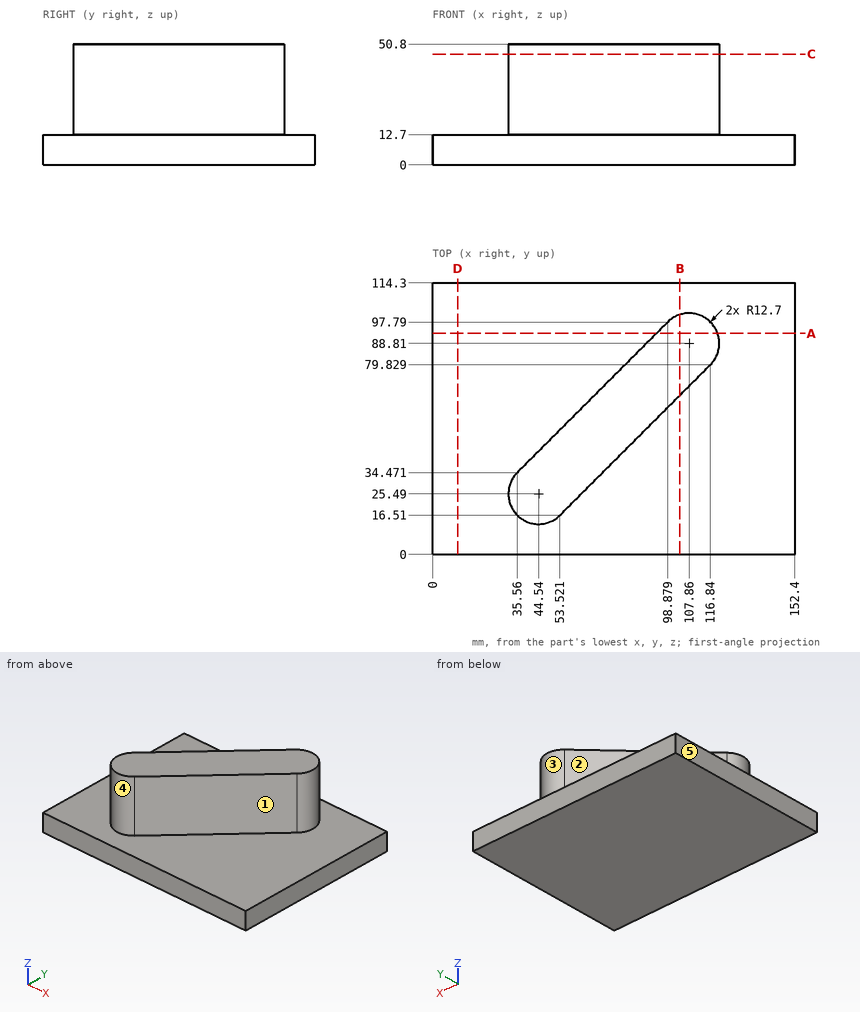
Job drawing, mm, ordinate dimensions from the low corner. One solid piece. A direction names the side the tool comes from. Round coordinates to 2 decimals unless told otherwise and drop trailing zeros. Order: outer loops, then holes, each group sorted by start corner. A loop starts at its lowest first (then second) coordinate and runs counter-clockwise, first axis right, second up. Notation, with made-up numbers: (42.25, 25) -> (67.25, 25) arc R33 ccw to (67.25, 58) -> close; hole circle Ø5 at (75, 52.25). An arc over 180 degrees is marked (long way). Write item = value, one per line.
(1) Cut at B-B (x = 104). Write the cut outline in (y, z).
Answers follow:
outline = (0, 0) -> (114.3, 0) -> (114.3, 12.7) -> (100.91, 12.7) -> (100.91, 50.8) -> (66.99, 50.8) -> (66.99, 12.7) -> (0, 12.7) -> close
(2) 3-axis set-ups, long thin cutter, end or side, ignore diameter. For the marked faces 4 and 5: which of +Z, -Z, +X, -X, +Y, -Y reach the whole face in a straight line?
Answers follow:
face_4 = +Z
face_5 = +Z, -Z, -X, +Y, -Y
(3) Cut at A-A (y = 93). Write the cut outline in (x, z), plus the area to 3 significant figures.
Answers follow:
outline = (0, 0) -> (152.4, 0) -> (152.4, 12.7) -> (119.85, 12.7) -> (119.85, 50.8) -> (94.09, 50.8) -> (94.09, 12.7) -> (0, 12.7) -> close
area = 2,920 mm²
(4) Drill centre lines: L1, parallel to Z at x = 28, y = 95; L2, parallel to X at y = 35.5, z = 17; L3, parallel to X at y = 67.5, z = 25. Where is each one in solid material? Low to high.
Answers follow:
L1 = 0 to 12.7
L2 = 36.59 to 72.51
L3 = 68.59 to 104.51
(5) Flat gauge pins, fed straight in: P1, Ø5, axis at y = 68.5, z = 33.5, coming from the +X side; P2, Ø4, axis at x = 95, z = 29, coming from the +Y side; P3, Ø8, axis at y = 65.5, z = 21, coming from the +X side. Where does each tip first touch, or does it go through?
Answers follow:
P1 = 108.01
P2 = 95.91
P3 = 106.51
(6) Cut at D-D (x = 10.5). Write the cut outline in (y, z).
Answers follow:
outline = (0, 0) -> (114.3, 0) -> (114.3, 12.7) -> (0, 12.7) -> close
(7) Cut at C-C (z = 46.5). Write the cut outline in (x, y), plus the area to 3 significant figures.
Answers follow:
outline = (35.56, 34.47) arc R12.7 ccw to (53.52, 16.51) -> (116.84, 79.83) arc R12.7 ccw to (98.88, 97.79) -> close
area = 2,780 mm²
(8) Pull direction X, two halves, no side cores. Call the marked faces 1, 2 and 3: +X half, -X half, draft (parallel to the pull), parting line (faces both ways), or undercut.
Answers follow:
face_1 = +X half
face_2 = -X half
face_3 = parting line
